Could you check a few things on this model? Use its own coordinates, in mm. Give positions to 0.01 mm unless a question says otherwise; leave off trailing zeros. Loops run counter-clockwise (first coordinate to the right, second up) from the corner with the lowest first, then second, coordinate; pieces in that order, holes last. Notation, with made-up numbers: M 52.5,58.5 L 93.5,58.5 A9 cw 93.5,64.5 Z; hole C 22.25,-2.75 d10. An arc over 180 degrees is marked long. Use CSV: the item, a comma, the result in double quotes.
```python
from build123d import *

# Parameters (mm, degrees)
SKETCH1_R           = 3.98145
SKETCH1_R_2         = 3.1877
BOSS_EXTRUDE1_DEPTH = 6.35


with BuildPart() as part:
    # Sketch1 → Boss-Extrude1 (new body)
    with BuildSketch(Plane(origin=(0, 0, 0), x_dir=(1, 0, 0), z_dir=(0, 1, 0))):
        with BuildLine():
            Line((0, 0), (10.0584, 0))
            Line((10.0584, 0), (22.635934302, 9.700812927))
            ThreePointArc((22.635934302, 9.700812927), (25.9334, 16.4084), (22.635934302, 23.115987073))
            Line((22.635934302, 23.115987073), (10.0584, 32.8168))
            Line((10.0584, 32.8168), (0, 32.8168))
            ThreePointArc((0, 32.8168), (-16.4084, 16.4084), (0, 0))
        make_face()
        with Locations(Location((0, 16.4084, 0), (0, 0, 270))):
            Circle(SKETCH1_R, mode=Mode.SUBTRACT)
        with Locations(Location((17.4625, 16.4084, 0), (0, 0, 270))):
            Circle(SKETCH1_R_2, mode=Mode.SUBTRACT)
    extrude(amount=BOSS_EXTRUDE1_DEPTH)


solid = part.part
```
1. I want a section at A-A, the plane x = -0.5. List the corners of the cut face in (y, z) for me.
Outcome:
outline,"M 0,-32.81 L 6.35,-32.81 L 6.35,-20.36 L 0,-20.36 Z; M 0,-12.46 L 6.35,-12.46 L 6.35,-0.01 L 0,-0.01 Z"
2. If we mould it in two halves opening along X, with no side actions, what happens to faces 1 (the face through (20.15, 3.131, -14.695)), 2 (the face through (5, 3, -32.817)), 3 (the face through (16.435, 3.131, -27.898))? For each: +X half, -X half, draft (parallel to the pull), parting line (faces both ways), or undercut.
Outcome:
face 1,"undercut"
face 2,"draft"
face 3,"+X half"
3. Please list where these lines run through material, in increasing order: line 1 (X direction, y = 6.25, z = -17); line 2 (X direction, y = 1, z = -16); line 3 (Z direction, x = 19.5, y = 4).
Outcome:
line 1,"-16.4 to -3.94, 3.94 to 14.33, 20.59 to 25.91"
line 2,"-16.4 to -3.96, 3.96 to 14.3, 20.62 to 25.92"
line 3,"-25.53 to -18.86, -13.96 to -7.28"
4. I want a section at C-C, the plane z = -6. List the corners of the cut face in (x, y) for me.
Outcome:
outline,"M -12.68,0 L 17.84,0 L 17.84,6.35 L -12.68,6.35 Z"
5. I'm going to push flat-ended pins straight in: pin 1 Ø2 at (x, y) = (13, 4.5) entering from +Z; pin 2 Ø3 at (x, y) = (13, 2.5) entering from +Z. Where does each tip first touch, or does it pass through?
Outcome:
pin 1,"z = -1.5"
pin 2,"z = -1.11"
6. I want a section at B-B, the plane y = 3. List the corners of the cut face in (x, z) for me, then the cut area to 3 significant figures.
Outcome:
outline,"M 0,-32.82 L 10.06,-32.82 L 22.64,-23.12 A8.47 ccw 22.64,-9.7 L 10.06,0 L 0,0 A16.41 ccw Z; hole C 0,-16.41 d7.96; hole C 17.46,-16.41 d6.38"
area,"993 mm2"
7. I want a section at D-D, the plane x = -12. List the corners of the cut face in (y, z) for me.
Outcome:
outline,"M 0,-27.6 L 6.35,-27.6 L 6.35,-5.22 L 0,-5.22 Z"
